```python
from build123d import *

# Parameters (mm, degrees)
F0_W     = 88.39527
F0_H     = 153.20968
F0_R     = 22.6744372739
F1_DEPTH = 5
F0_W_2   = 9.8689098377
F0_H_2   = 3.4395875409
F0_W_3   = 9.86891
F0_H_3   = 3.43959
F2_DEPTH = 3.9
F3_DEPTH = 25
F4_R     = 3.8627416998
F5_SIZE  = 2.5


# Not quite as in the source:
# - a feature names something its author has since deleted; it is built from what else it names


with BuildPart() as f1:
    # F0 (on Front) → F1 (new body)
    with BuildSketch(Plane.XZ):
        with Locations((4.9840081745, 0.7166508444)):
            Rectangle(F0_W, F0_H)
        with Locations((4.9144495279, -0.1638149843)):
            Circle(F0_R, mode=Mode.SUBTRACT)
    extrude(amount=F1_DEPTH)

    # F0 (on Front) → F2 (join)
    with BuildSketch(Plane.XZ):
        with Locations((4.9144495279, -0.1638149843)):
            Circle(F0_R)
        with Locations((3.791642841, -9.5432697745)):
            Rectangle(F0_W_2, F0_H_2, mode=Mode.SUBTRACT)
        with Locations((-2.0837161803, 0.0662026977)):
            Rectangle(F0_W_3, F0_H_3, mode=Mode.SUBTRACT)
        with BuildLine():
            Line((18.1140358327, 2.2190151321), (18.1140358327, -2.0737481719))
            Line((18.1140358327, -2.0737481719), (14.117325074, -2.0737481719))
            ThreePointArc((14.117325074, -2.0737481719), (11.9709434221, 0.0726334801), (14.117325074, 2.2190151321))
            Line((14.117325074, 2.2190151321), (18.1140358327, 2.2190151321))
        make_face(mode=Mode.SUBTRACT)
        with Locations((3.791642841, 9.6756751699)):
            Rectangle(F0_W_2, F0_H_2, mode=Mode.SUBTRACT)
    extrude(amount=F2_DEPTH)

    # F0 (on Front) → F3 (join)
    with BuildSketch(Plane.XZ):
        with Locations((3.791642841, -9.5432697745)):
            Rectangle(F0_W_2, F0_H_2)
        with Locations((-2.0837161803, 0.0662026977)):
            Rectangle(F0_W_3, F0_H_3)
        with Locations((3.791642841, 9.6756751699)):
            Rectangle(F0_W_2, F0_H_2)
        with BuildLine():
            Line((14.117325074, -2.0737481719), (18.1140358327, -2.0737481719))
            Line((18.1140358327, -2.0737481719), (18.1140358327, 2.2190151321))
            Line((18.1140358327, 2.2190151321), (14.117325074, 2.2190151321))
            ThreePointArc((14.117325074, 2.2190151321), (11.9709434221, 0.0726334801), (14.117325074, -2.0737481719))
        make_face()
    extrude(amount=F3_DEPTH)

    # F4
    f4_edges = [f1.edges().sort_by_distance(p)[0] for p in [
        (-1.142812, -25, -9.54327),
        (8.726098, -25, -9.54327),
        (-7.018171, -25, 0.066203),
        (2.850739, -25, 0.066203),
        (8.726098, -25, 9.675675),
        (-1.142812, -25, 9.675675),
    ]]
    fillet(f4_edges, radius=F4_R)

    # F5
    f5_edges = [f1.edges().sort_by_distance(p)[0] for p in [
        (18.114036, -25, 0.072633),
    ]]
    chamfer(f5_edges, length=F5_SIZE)


solid = f1.part
```
Verification items for the finished model (mm, model axes). A direction names the side the tool comes from. Round coordinates to 2 decimals unless told otherwise and drop trailing zeros. Write each loop counter-clockwise with the first axis right and the second up, starting at its lowest first coordinate (ties: lowest second). Pieces come first, ordered by that corner, then holes. Notation, with made-up numbers: (33, 69.25) - (70, 69.25) arc R12 cw to (70, 87.25) - close; hole circle Ø4 at (37, 17). An arc over 180 degrees is marked (long way). Answer as a JSON object with one key per item and string values. Group by question number.
Q1. Go/stop test with flat-tipped pins: pin 1 Ø3 at (y, z) = (-13.5, -10) entering from +X; pin 2 Ø2 at (x, y) = (15, -10) entering from +Z; pin 3 Ø1 at (x, z) = (29.5, 27) entering from -Y. Record where each tip stops, or that it passes through.
Q2. Section check C-C, the plane z = 60. Enter the section's corners in (x, y).
Q3. Section check B-B, the plane x = 23.5. Enter the section's corners in (y, z).
Q4. Section check D-D, the plane z = 16. Enter the section's corners in (x, y).
Q5. Thickness scan on line 1 (Z direction, x = 2.5, y = -5.5); line 2 (Y direction, x = -32, z = -7.5); line 3 (Z direction, x = 7, y = -17). Record the ranges inside material, lowest first.
Q6. Mould release check, pull along X, two halves, no side actions. Record for faces 1 (the cylindrical face through (1.75, -23.84, 0.09)), 2 (the cylindrical face through (-5.917, -23.838, 0.09)), 3 (the flat face through (4, -2, 77.321)): released by +X, released by -X, zero draft, split by the parting line, or undercut.
Q7. Section check A-A, the plane y = -7.75. Enter the section's corners in (x, z).
Q8. Tool access check on faces 4 (the cylindrical face through (-0.04, -23.84, 9.7)), 5 (the cylindrical face through (0, -4.4, -22.3)), 6 (the cylindrical face through (7.565, -23.898, -9.519)), 7 (the cylindrical face through (-0.04, -23.84, -9.52)). Record the directions out of +Z, -Z, +X, -X, +Y, -Y that give a thin tool (end or side, any length) a straight path to the whole face; none if there is none.
Found:
{
 "1": {"pin 1": "stops at x = 8.73", "pin 2": "stops at z = 2.22", "pin 3": "stops at y = -5"},
 "2": {"outline": "(-39.21, -5) - (49.18, -5) - (49.18, 0) - (-39.21, 0) - close"},
 "3": {"outline": "(-5, -75.89) - (0, -75.89) - (0, 77.32) - (-5, 77.32) - (-5, 12.82) - (-3.9, 12.82) - (-3.9, -13.15) - (-5, -13.15) - close"},
 "4": {"outline": "(-39.21, -5) - (-10.99, -5) - (-10.99, -3.9) - (20.82, -3.9) - (20.82, -5) - (49.18, -5) - (49.18, 0) - (-39.21, 0) - close"},
 "5": {"line 1": "z = -11.26 to -7.82, -1.65 to 1.79, 7.96 to 11.4", "line 2": "y = -5 to 0", "line 3": "z = -11.26 to -7.82, 7.96 to 11.4"},
 "6": {"face 1": "undercut", "face 2": "released by -X", "face 3": "zero draft"},
 "7": {"outline": "(-7.02, -1.65) - (2.85, -1.65) - (2.85, 1.79) - (-7.02, 1.79) - close; (-1.14, -11.26) - (8.73, -11.26) - (8.73, -7.82) - (-1.14, -7.82) - close; (-1.14, 7.96) - (8.73, 7.96) - (8.73, 11.4) - (-1.14, 11.4) - close; (14.12, -2.07) - (18.11, -2.07) - (18.11, 2.22) - (14.12, 2.22) arc R2.15 ccw to start"},
 "8": {"face 4": "+Z, -X, -Y", "face 5": "-Y", "face 6": "+Z, -Z, +X, -Y", "face 7": "-Z, -X, -Y"}
}
